Verification items for this drawing (mm, ordinates from the low corner). A direction names the side the tool comes from. Round coordinates to 2 decimals unless told otherwise and drop trailing zeros. Loops run counter-clockwise (first coordinate to the right, second up) from the corner with the lowest first, then second, coordinate; pieces in that order, holes last. Notation, with made-up numbers: (-6.75, -16) - (29.25, -16) arc R25 cw to (29.25, 12) - close; hole circle Ø2 at (-14, 11). An arc over 180 degrees is marked (long way). Put each result on its own line as item: value.
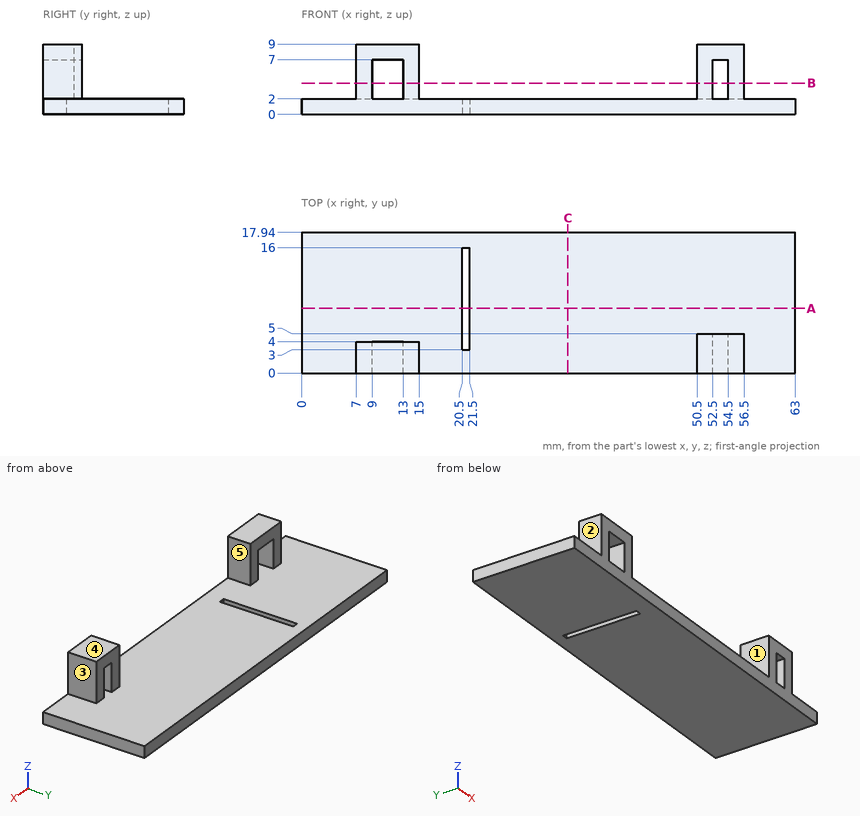
Item 1: Release check for a two-part mould opening along X. For the marked faces 1, 2 and 3 record: +X half, -X half, draft (parallel to the pull), parting line (faces both ways), or undercut.
Filled sheet:
face 1: undercut
face 2: -X half
face 3: +X half
Item 2: Section check B-B on z = 4. Enter the section's corners in (x, y).
Filled sheet:
outline: (7, 0) - (9, 0) - (9, 4) - (7, 4) - close; (13, 0) - (15, 0) - (15, 4) - (13, 4) - close; (50.5, 0) - (52.5, 0) - (52.5, 5) - (50.5, 5) - close; (54.5, 0) - (56.5, 0) - (56.5, 5) - (54.5, 5) - close
Item 3: Section check A-A on y = 8.25. Enter the section's corners in (x, z).
Filled sheet:
outline: (0, 0) - (20.5, 0) - (20.5, 2) - (0, 2) - close; (21.5, 0) - (63, 0) - (63, 2) - (21.5, 2) - close
Item 4: Go/stop test with flat-tipped pins: pin 1 (4.5 mm diameter, centred on y = 2.5, z = 4.5, fed in from -X); pin 2 (10 mm diameter, centred on x = 36.5, y = 7, fed in from +Z); pin 3 (2 mm diameter, centred on y = 2.5, z = 6.5, fed in from +X). Record where each tip stops, or that it passes through.
Filled sheet:
pin 1: x = 7
pin 2: z = 2
pin 3: x = 56.5
Item 5: Section check C-C on x = 34. Enter the section's corners in (y, z), then the cut area to 3 significant figures.
Filled sheet:
outline: (0, 0) - (17.94, 0) - (17.94, 2) - (0, 2) - close
area: 35.9 mm²
Item 6: Thickness scan on line 1 (X direction, y = 1.5, z = 4); line 2 (X direction, y = 9, z = 0.75); line 3 (Z direction, x = 11, y = 12.5). Record the ranges inside material, lowest first. Write a range as from..to.
Filled sheet:
line 1: 7..9, 13..15, 50.5..52.5, 54.5..56.5
line 2: 0..20.5, 21.5..63
line 3: 0..2
Item 7: Tool access check on the marked faces 4 and 5. Record the directions out of +Z, -Z, +X, -X, +Y, -Y that give a thin tool (end or side, any length) a straight path to the whole face; none if there is none.
Filled sheet:
face 4: +Z, +X, -X, +Y, -Y
face 5: +Z, +Y, -Y
